For this review, take the finished solid that the model builds, in its own axes (mm). Give positions to 0.01 mm unless a question says otherwise; leave off trailing zeros. Order: outer loops, then holes, each group sorted by start corner. A loop starts at its lowest first (then second) coordinate and runs counter-clockwise, first axis right, second up. Notation, with made-up numbers: (-34.5, 67) - (18.5, 67) arc R24 ccw to (18.5, 78) - close; hole circle Ø1 at (-17, 22). An arc over 180 degrees is marked (long way). Use a Markdown table: item, result. Add a question column.
1) Wall thickness on L1, parallel to Y at x = 40, z = 2.75; L2, parallel to X at y = 183, z = 2.7; L3, parallel to X at y = 119.5, z = 1.5: over which ranges is each line inside the solid? List them lowest first.
2) We need section B-B on y = 183. Write out the cut boundary in (x, z).
3) We need section A-A on x = 40. Write out the cut boundary in (y, z), then the cut area to 3 significant figures.
4) Clearance check with flat-ended pins moving along their axes: P1, Ø1.5, axis at x = 115, z = 3.5, coming from the -Y side; P2, Ø2, axis at y = 156.5, z = 2, coming from the -X side; P3, Ø1.5, axis at x = 88, y = 119.5, coming from the -Z side; P4, Ø1.2, axis at x = 178.5, z = 2.5, coming from the +Y side. State where each tip first meets the part, or that it passes through.
5) We need section D-D on y = 126. Write out the cut boundary in (x, z).
6) Mouldability with a two-part tool opening along X and no side actions: class faces 1 (the face through (90, 74, 4)), 2 (the face through (37.2, 180.9, 2)) as released by +X, released by -X, zero draft, split by the parting line, or undercut.
7) We need section C-C on z = 1.1. Give the number of separate pieces and of enclosed holes in the cut face, then the cut area to 3 significant figures.
```python
from build123d import *

# Parameters (mm, degrees)
SKETCH_1_W      = 30.4
SKETCH_1_H      = 4.4
SKETCH_1_W_2    = 4.4
SKETCH_1_H_2    = 20.4
SKETCH_1_R      = 3.5
EXTRUDE_1_DEPTH = 4


with BuildPart() as part:
    # Эскиз1 → Бобышка-Вытянуть1 (new body)
    with BuildSketch(Plane.XY):
        Polygon((0, 20), (0, 0), (26.99543951, 0), (26.99543951, -4), (56.99543951, -4), (56.99543951, 0), (136.99543951, 0), (136.99543951, -4), (166.99543951, -4), (166.99543951, 0), (187, 0), (187, 133), (50, 133), (50, 193), (30, 193), (30, 133), (0, 133), (0, 120), (-4, 120), (-4, 100), (0, 100), (0, 40), (-4, 40), (-4, 20), align=None)
        with Locations((43.5, 67.2)):
            Rectangle(SKETCH_1_W, SKETCH_1_H, mode=Mode.SUBTRACT)
        with Locations((179, 38)):
            Rectangle(SKETCH_1_W_2, SKETCH_1_H_2, mode=Mode.SUBTRACT)
        with Locations((143.5, 67.2)):
            Rectangle(SKETCH_1_W, SKETCH_1_H, mode=Mode.SUBTRACT)
        with Locations((179, 113.2)):
            Rectangle(SKETCH_1_W_2, SKETCH_1_H_2, mode=Mode.SUBTRACT)
        with Locations((40, 183)):
            Circle(SKETCH_1_R, mode=Mode.SUBTRACT)
    extrude(amount=EXTRUDE_1_DEPTH)


solid = part.part
```
Checked values:
| question | item | result |
|---|---|---|
| 1 | L1 | -4 to 65, 69.4 to 179.5, 186.5 to 193 |
| 1 | L2 | 30 to 36.5, 43.5 to 50 |
| 1 | L3 | -4 to 176.8, 181.2 to 187 |
| 2 | outline | (30, 0) - (36.5, 0) - (36.5, 4) - (30, 4) - close; (43.5, 0) - (50, 0) - (50, 4) - (43.5, 4) - close |
| 3 | outline | (-4, 0) - (65, 0) - (65, 4) - (-4, 4) - close; (69.4, 0) - (179.5, 0) - (179.5, 4) - (69.4, 4) - close; (186.5, 0) - (193, 0) - (193, 4) - (186.5, 4) - close |
| 3 | area | 742 mm² |
| 4 | P1 | y = 0 |
| 4 | P2 | x = 30 |
| 4 | P3 | z = 0 |
| 4 | P4 | y = 133 |
| 5 | outline | (0, 0) - (187, 0) - (187, 4) - (0, 4) - close |
| 6 | face 1 | zero draft |
| 6 | face 2 | undercut |
| 7 | separate pieces | 1 |
| 7 | enclosed holes | 5 |
| 7 | area | 26,000 mm² |
